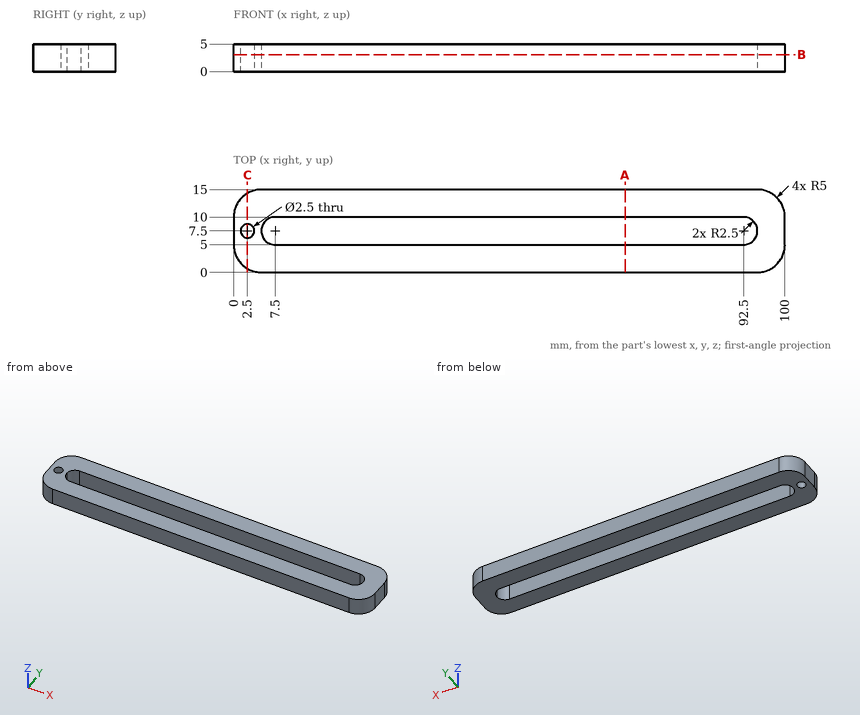
For this review, use the dimensioned drawing (mm, ordinates from the lowest corner) and the shaded views. Give positions to 0.01 mm unless a question says otherwise; leave off trailing zeros. Write each loop counter-clockwise with the first axis right and the second up, starting at its lowest first coordinate (ties: lowest second). Pieces come first, ordered by that corner, then holes. Notation, with made-up numbers: M -16,-28.5 L 14,-28.5 A12 cw 14,-17.5 Z; hole C 44,31 d9. An arc over 180 degrees is marked long. Answer as a JSON object with one key per item and string values. Group by question number.
Item 1: Consider section B-B on z = 3.05. Write out the cut boundary in (x, y).
Item 2: Consider section A-A on x = 71. Write out the cut boundary in (y, z), plus the area to 3 significant figures.
Item 3: Consider section C-C on x = 2.5. Write out the cut boundary in (y, z).
Item 4: For pin 1 Ø1.5 at (x, y) = (2.5, 7.5) entering from +Z, flat-tipped, find the tip position at first contact; note if it passes through.
Item 5: For probe 1 along Y at (x, z) = (20.5, 2.35); probe 2 along Y at (x, z) = (2.5, 1.45); probe 3 along X at (y, z) = (10.5, 1.25), list the stretches that pass through material, from the lowest coordinate up. Write a range as [from, to].
Check result:
{
 "1": {"outline": "M 0,5 A5 ccw 5,0 L 95,0 A5 ccw 100,5 L 100,10 A5 ccw 95,15 L 5,15 A5 ccw 0,10 Z; hole C 2.5,7.5 d2.5; hole M 7.5,5 L 92.5,5 A2.5 ccw 92.5,10 L 7.5,10 A2.5 ccw Z"},
 "2": {"outline": "M 0,0 L 5,0 L 5,5 L 0,5 Z; M 10,0 L 15,0 L 15,5 L 10,5 Z", "area": "50.0 mm^2"},
 "3": {"outline": "M 0.67,0 L 6.25,0 L 6.25,5 L 0.67,5 Z; M 8.75,0 L 14.33,0 L 14.33,5 L 8.75,5 Z"},
 "4": {"pin 1": "passes through"},
 "5": {"probe 1": "y = [0, 5], [10, 15]", "probe 2": "y = [0.67, 6.25], [8.75, 14.33]", "probe 3": "x = [0.03, 99.97]"}
}
